Geometry: final body of the model. Coordinates: model frame, mm. Coordinates: 2 decimals unless noted, no trailing zeros. Order: outer loops, then holes, each group sorted by start corner. A loop starts at its lowest first (then second) coordinate and runs counter-clockwise, first axis right, second up. Notation, with made-up numbers: (-33.75, 60.25) - (-6.75, 60.25) arc R23 cw to (-6.75, 97.25) - close; hole circle Ø5 at (69.5, 73). An arc over 180 degrees is marked (long way). Use a Markdown table: item, result. Add a question column.
Autodesk Inventor part; units mm, degrees
ref_plane "YZ Plane" through (0, 0, 0) normal (1, 0, 0) x (0, 1, 0)
ref_plane "XZ Plane" through (0, 0, 0) normal (0, 1, 0) x (-1, 0, 0)
ref_plane "XY Plane" through (0, 0, 0) normal (0, 0, 1) x (1, 0, 0)
sketch "Sketch1" plane through (0, 0, 0) normal (0, 0, 1) x (1, 0, 0)
  circle A0 centre (0, 0) radius 25
  dimension "d0" = 50
extrude "Extrusion1" add sketch "Sketch1" along normal blind 2000
sketch "Sketch2" plane through (0, 0, 2000) normal (0, 0, 1) x (1, 0, 0)
  circle A0 centre (0, 0) radius 23
  dimension "d3" = 46
extrude "Extrusion2" cut sketch "Sketch2" against normal blind 2000
sketch "Sketch3" plane through (0, 0, 0) normal (1, 0, 0) x (0, 1, 0)
  circle A0 centre (0, 1970) radius 4.5
  line L0 (25, 2000) -> (-25, 2000)
  point P0 (0, 0)
  dimension "d6" = 9
  dimension "d7" = 30
extrude "Extrusion3" cut sketch "Sketch3" along normal through all both and the other way through all
properties part number "Odnogi"
1) Section A-A (x = 0). Return loops of the section in (y, z).
2) Ray query, line 1 along X through (y, z) = (0, 1073); line 2 along Y through (x, z) = (4, 652). Return the intervals inside material, ascending.
3) Section C-C (z = 344.5). Return loops of the section in (x, y), then the cut area to 3 significant figures.
4) Section B-B (y = -15). Return loops of the section in (x, z).
5) Draft query along X for faces 1 (the face through (-2.994, 22.804, 1014)), 2 (the face through (22.1, -7.3, 0)), 3 (the face through (11.5, 22.2, 986)). Return one class per face: pulls with the +X half, pulls with the -X half, needs draft (parallel to the pull), parting line crosses it, or undercut.
6) Pin query (flat end, axial travel): pin 1 (4 mm diameter, centred on x = -17, z = 300.5, fed in from -Y); pin 2 (1 mm diameter, centred on y = 15, z = 1196.5, fed in from -X); pin 3 (1.5 mm diameter, centred on x = -8, z = 510, fed in from -Y). Return the tip coordinate at first contact, or that it passes through.
Values follow:
| question | item | result |
|---|---|---|
| 1 | outline | (-25, 0) - (-23, 0) - (-23, 2000) - (-25, 2000) - close; (23, 0) - (25, 0) - (25, 2000) - (23, 2000) - close |
| 2 | line 1 | x = -25 to -23, 23 to 25 |
| 2 | line 2 | y = -24.68 to -22.65, 22.65 to 24.68 |
| 3 | outline | circle Ø50 at (0, 0); hole circle Ø46 at (0, 0) |
| 3 | area | 302 mm² |
| 4 | outline | (-20, 0) - (-17.44, 0) - (-17.44, 2000) - (-20, 2000) - close; (17.44, 0) - (20, 0) - (20, 2000) - (17.44, 2000) - close |
| 5 | face 1 | undercut |
| 5 | face 2 | needs draft |
| 5 | face 3 | parting line crosses it |
| 6 | pin 1 | stops at y = -20 |
| 6 | pin 2 | stops at x = -20.37 |
| 6 | pin 3 | stops at y = -23.93 |
